Autodesk Inventor part; units mm, degrees
ref_plane "YZ Plane" through (0, 0, 0) normal (1, 0, 0) x (0, 1, 0)
ref_plane "XZ Plane" through (0, 0, 0) normal (0, 1, 0) x (-1, 0, 0)
ref_plane "XY Plane" through (0, 0, 0) normal (0, 0, 1) x (1, 0, 0)
sketch "Sketch4" plane through (0, 0, 0) normal (0, 1, 0) x (-1, 0, 0)
  line L0 (99, -200) -> (-99, -200)
  line L1 (-99, -200) -> (-99, 200)
  line L2 (-99, 200) -> (99, 200)
  line L3 (99, 200) -> (99, -200)
  line L4 (99, -200) -> (-99, 200) construction
  point P0 (0, 0)
  point P1 (0, 0)
  dimension "d24" = 198
  dimension "d25" = 400
extrude "Plate4" add sketch "Sketch4" along normal mid plane 2
sketch "Sketch7" plane through (0, -1, 0) normal (0, -1, 0) x (1, 0, 0)
  circle A0 centre (48, 75) radius 5
  line L0 (99, 200) -> (99, -200)
  line L1 (99, -200) -> (-99, -200)
  line L2 (0, -200) -> (0, 200) construction
  line L3 (99, 0) -> (-99, 0) construction
  circle A1 centre (-48, 75) radius 5
  circle A2 centre (48, 160) radius 5
  circle A3 centre (-48, 160) radius 5
  line L4 (99, 200) -> (-99, 200)
  point P0 (0, 0)
  point P1 (0, 0)
  dimension "d41" = 10
  dimension "d46" = 85
  dimension "d57" = 96
  dimension "d70" = 125
extrude "Extrusion2" cut sketch "Sketch7" against normal up to surface (2 mm away)
sketch "Sketch9" plane through (97, 1, -200) normal (1, 0, 0) x (0, -1, 0)
  line L0 (0, 400) -> (0, 0)
  line L1 (0, 0) -> (25, 0)
  line L2 (25, 0) -> (25, 400)
  line L3 (25, 400) -> (0, 400)
edge flange "Flange5" height 25 angle 90 thickness 2 bend radius 2 thickness toward (1, 0, 0) relief tear relief width 2 relief depth 1 corner gap 2 corner form 0 edges at (99, 1, 0) (-99, 1, 0) wall of the first edge with corners at (97, 1, 200) (97, 1, -200) (97, -24, -200) (97, -24, 200)
bend "Bend5"
corner "Corner5"
equation "\"d24\" = Ширина_базовой_пластины"
equation "\"d25\" = Длина_базовой_пластины"
equation "\"d26\" = Thickness"
equation "\"d60\" = BendReliefWidth"
equation "\"d61\" = BendReliefDepth"
equation "\"d62\" = MinimumRemnant"
equation "\"d63\" = TransitionRadius"
equation "\"d66\" = BendRadius"
equation "\"d67\" = CornerReliefSize"
equation "\"d68\" = GapSize"
equation "\"d69\" = JacobiRadiusSize"
equation "\"BendRadius\" = Thickness"
equation "\"BendReliefWidth\" = Thickness"
equation "\"BendReliefDepth\" = 0.5 * Thickness"
equation "\"CornerReliefSize\" = 4 * Thickness"
equation "\"MinimumRemnant\" = 2 * Thickness"
equation "\"TransitionRadius\" = BendRadius"
equation "\"JacobiRadiusSize\" = BendRadius"
equation "\"GapSize\" = Thickness"
properties part number "Крепление"
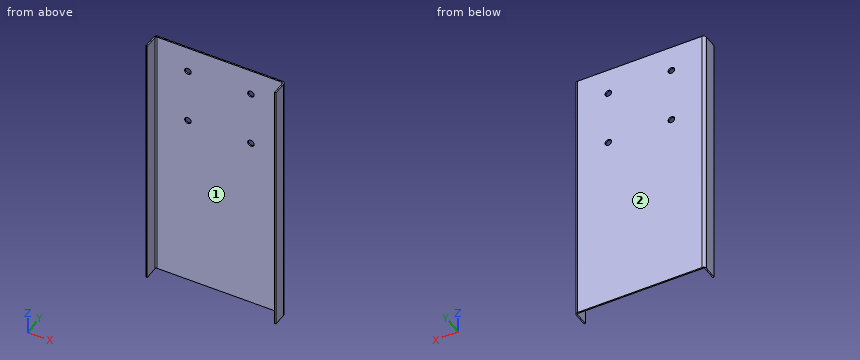
Part model, mm, in its own coordinate system. Face numbers are marked on the shaded views. Give positions to 0.01 mm unless a question says otherwise; leave off trailing zeros. Order: outer loops, then holes, each group sorted by start corner. A loop starts at its lowest first (then second) coordinate and runs counter-clockwise, first axis right, second up. Notation, with made-up numbers: M -37.5,66 L -1.5,66 A33 cw -1.5,100 Z; hole C 72,50.5 d2. An arc over 180 degrees is marked long. Use a Markdown table: item, result. Add a question column.
(1) Mould opens along X. For the marked faces 1 and 2 say: +X half, -X half, draft (parallel to the pull), parting line (faces both ways), or undercut.
(2) Saw through at A-A, the plane z = 75. Give the cut face in (x, y), and give its area (3 significant figures).
(3) Saw through at C-C, the plane y = -9.5. Give the cut face in (x, z), and give its area (3 significant figures).
(4) Saw through at B-B, the plane x = 48. Give the cut face in (y, z).
(5) Probe line 1 along Z through (x, y) = (48, -0.1); line 2 along X through (y, z) = (-11, -171.5); line 3 along Y through (x, z) = (81.5, 32.5). List the from-to ranges inside material, lowest first. Write a range as [from, to].
(6) Drop a flat-ended pin along its axis: P1, Ø11.5, axis at x = 48, z = 75, coming from the -Y side. Give the stop position or say it passes through.
(7) Saw through at D-D, the plane z = 10. Give the cut face in (x, y), and give its area (3 significant figures).
Answer key:
| question | item | result |
|---|---|---|
| 1 | face 1 | undercut |
| 1 | face 2 | draft |
| 2 | outline | M -99,-24 L -97,-24 L -97,-3 A2 cw -95,-1 L -53,-1 L -53,1 L -95,1 A4 ccw -99,-3 Z; M -43,-1 L 43,-1 L 43,1 L -43,1 Z; M 53,-1 L 95,-1 A2 cw 97,-3 L 97,-24 L 99,-24 L 99,-3 A4 ccw 95,1 L 53,1 Z |
| 2 | area | 443 mm^2 |
| 3 | outline | M -99,-200 L -97,-200 L -97,200 L -99,200 Z; M 97,-200 L 99,-200 L 99,200 L 97,200 Z |
| 3 | area | 1,600 mm^2 |
| 4 | outline | M -1,-200 L 1,-200 L 1,70 L -1,70 Z; M -1,80 L 1,80 L 1,155 L -1,155 Z; M -1,165 L 1,165 L 1,200 L -1,200 Z |
| 5 | line 1 | [-200, 70], [80, 155], [165, 200] |
| 5 | line 2 | [-99, -97], [97, 99] |
| 5 | line 3 | [-1, 1] |
| 6 | P1 | y = -1 |
| 7 | outline | M -99,-24 L -97,-24 L -97,-3 A2 cw -95,-1 L 95,-1 A2 cw 97,-3 L 97,-24 L 99,-24 L 99,-3 A4 ccw 95,1 L -95,1 A4 ccw -99,-3 Z |
| 7 | area | 483 mm^2 |
